Input: part model. Units: mm. Frame: model coordinates. Face numbers are marked on the shaded views. A direction names the side the tool comes from. Round coordinates to 2 decimals unless told otherwise and drop trailing zeros. Loops run counter-clockwise (first coordinate to the right, second up) from the corner with the lowest first, then second, coordinate; pieces in that order, holes last.
(1) Access query for the marked faces 1, 2 and 3. Directions: +Z, -Z, +X, -X, +Y, -Y. A direction counts if a zero-diameter tool reaches every point of the face in a straight line with its end or side. Return the directions, or none.
(2) Cut plane B-B, the plane y = 15. Output: boundary loops of the cut face in (x, z) (1 decimal), and give its area (3 significant figures).
(3) Cut plane C-C, the plane y = 3.5. Output: boundary loops of the cut face in (x, z).
(4) Cut plane A-A, the plane y = 9. Output: boundary loops of the cut face in (x, z) (1 decimal).
(5) First-contact query: pin 1 Ø1 at (y, z) = (3.5, -2) entering from -X; pin 2 Ø7 at (x, z) = (0, 0) entering from -Y; pin 3 Ø1.5 at (x, z) = (-1.5, 5.5) entering from +Y; pin 4 Ø1 at (y, z) = (16, -2.5) entering from +X. Flat tips, straight axial feed; report the tip coordinate or a pass-through.
(6) Draft query along Z for the marked faces 4, 5 and 6. Return one class per face: released by +Z, released by -Z, zero draft, split by the parting line, or undercut.
(7) Line query: line 1 (Z direction, x = -0.25, y = 13.25); line 2 (Z direction, x = 0, y = 4); line 3 (X direction, y = 13.75, z = 1.75). Output: solid intervals per line, ascending.
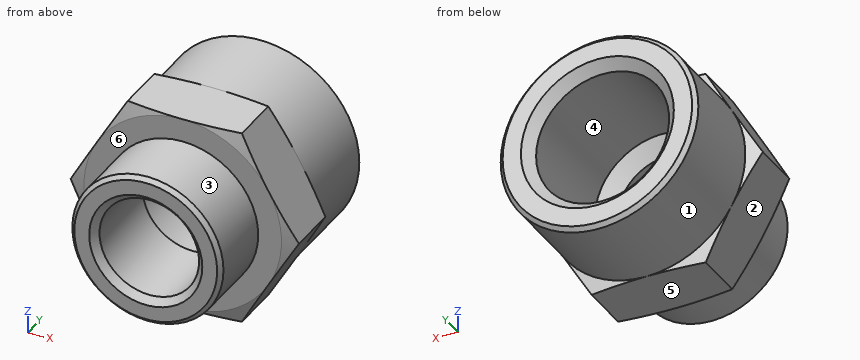
Autodesk Inventor part; units mm, degrees
ref_plane "ANBAU_XY" through (0, 7.5, 0) normal (0, 1, 0) x (1, 0, 0)
ref_plane "ANBAU_YZ" through (0, 7.5, 0) normal (1, 0, 0) x (0, 0, -1)
ref_plane "ANBAU_ZX" through (0, 7.5, 0) normal (0, 0, -1) x (0, 1, 0)
sketch "Sketch_12" plane through (0, 0, 0) normal (0, 0, 1) x (1, 0, 0)
  line L0 (0, 0) -> (0, 19)
  line L1 (0, 19) -> (8.1464, 19)
  line L2 (8.1464, 19) -> (8.5, 18.6464)
  line L3 (8.5, 18.6464) -> (8.5, 11)
  line L4 (8.5, 11) -> (10.2, 10.5445)
  line L5 (10.2, 10.5445) -> (10.2, 6.4555)
  line L6 (10.2, 6.4555) -> (8.5, 6)
  line L7 (8.5, 6) -> (6.5, 6)
  line L8 (6.5, 6) -> (6.5, 0.3536)
  line L9 (6.5, 0.3536) -> (6.1464, 0)
  line L10 (6.1464, 0) -> (0, 0)
  line L11 (0, 0) -> (0, 19)
revolve "Revolution1" add sketch "Sketch_12" angle 360 about axis through (0, 0, 0) along (0, -1, 0)
sketch "Sketch_13" plane through (0, 0, 0) normal (0, 1, 0) x (-1, 0, 0)
  line L0 (17, 17) -> (-17, 17)
  line L1 (-17, 17) -> (-17, -17)
  line L2 (-17, -17) -> (17, -17)
  line L3 (17, -17) -> (17, 17)
  line L4 (9.815, 0) -> (4.9075, 8.5)
  line L5 (4.9075, 8.5) -> (-4.9075, 8.5)
  line L6 (-4.9075, 8.5) -> (-9.815, 0)
  line L7 (-9.815, 0) -> (-4.9075, -8.5)
  line L8 (-4.9075, -8.5) -> (4.9075, -8.5)
  line L9 (4.9075, -8.5) -> (9.815, 0)
extrude "Extrusion1" cut sketch "Sketch_13" along normal blind 13.3
sketch "Sketch_14" plane through (0, 0, 0) normal (0, 0, 1) x (1, 0, 0)
  line L0 (0, 0) -> (0, 19)
  line L1 (0, 19) -> (6.5785, 19)
  line L2 (6.5785, 19) -> (5.7225, 18.144)
  line L3 (5.7225, 18.144) -> (5.7225, 8.55)
  line L4 (5.7225, 8.55) -> (4.283, 7.6)
  line L5 (4.283, 7.6) -> (4.283, 0.581)
  line L6 (4.283, 0.581) -> (4.864, 0)
  line L7 (4.864, 0) -> (0, 0)
  line L8 (0, 0) -> (0, 19)
revolve "Revolution2" cut sketch "Sketch_14" angle 360 about axis through (0, 0, 0) along (0, -1, 0)
thread "Thread1"
thread "Thread2"
ref_plane "ANBAU_XY" through (0, 7.5, 0) normal (0, 1, 0) x (1, 0, 0)
ref_plane "ANBAU_YZ" through (0, 7.5, 0) normal (1, 0, 0) x (0, 0, -1)
ref_plane "ANBAU_ZX" through (0, 7.5, 0) normal (0, 0, -1) x (0, 1, 0)
ref_plane "DICHTRING_XY" through (0, 9.5, 0) normal (0, 1, 0) x (1, 0, 0)
ref_plane "DICHTRING_YZ" through (0, 9.5, 0) normal (1, 0, 0) x (0, 0, -1)
ref_plane "DICHTRING_ZX" through (0, 9.5, 0) normal (0, 0, -1) x (0, 1, 0)
ref_plane "IP1_XY" through (0, 19, 0) normal (0, -1, 0) x (1, 0, 0)
ref_plane "IP1_YZ" through (0, 19, 0) normal (1, 0, 0) x (0, 0, 1)
ref_plane "IP1_ZX" through (0, 19, 0) normal (0, 0, 1) x (0, -1, 0)
ref_plane "IP2_XY" through (0, 9.5, 0) normal (0, 1, 0) x (1, 0, 0)
ref_plane "IP2_YZ" through (0, 9.5, 0) normal (1, 0, 0) x (0, 0, -1)
ref_plane "IP2_ZX" through (0, 9.5, 0) normal (0, 0, -1) x (0, 1, 0)
properties part number "8069220 NPFC-R-G14-G18-F"
Reported:
1. face 1: +Y
1. face 2: -Z, -X, +Y, -Y
1. face 3: -Y
2. outline: circle Ø17 at (0, 0); hole circle Ø11.4 at (0, 0)
2. area: 124 mm2
3. outline: circle Ø13 at (0, 0); hole circle Ø8.57 at (0, 0)
4. outline: (-9.8, 0) - (-4.9, -8.5) - (4.9, -8.5) - (9.8, 0) - (4.9, 8.5) - (-4.9, 8.5) - close; hole circle Ø11.4 at (0, 0)
5. pin 1: stops at x = -6.32
5. pin 2: passes through
5. pin 3: stops at y = 18.87
5. pin 4: stops at x = 8.26
6. face 4: undercut
6. face 5: released by -Z
6. face 6: zero draft
7. line 1: z = -8.5 to -5.72, 5.72 to 8.5
7. line 2: z = -6.5 to -4.28, 4.28 to 6.5
7. line 3: x = -8.32 to -5.45, 5.45 to 8.32
